from build123d import *

# Parameters (mm, degrees)
PAD_DEPTH    = 10
SKETCH001_R  = 16
POCKET_DEPTH = 3


with BuildPart() as part:
    # Sketch → Pad (new body)
    with BuildSketch(Plane.XY):
        with BuildLine():
            Line((-19, 70.33521), (19, 70.33521))
            Line((19, 70.33521), (19, -59.66479))
            ThreePointArc((-19, -59.66479), (0, -76.095918), (19, -59.66479))
            Line((-19, -59.66479), (-19, 70.33521))
        make_face()
    extrude(amount=PAD_DEPTH)

    # Sketch001 → Pocket (cut)
    with BuildSketch(Plane.XY.offset(10)):
        with Locations((0, 51.243999)):
            Circle(SKETCH001_R)
    extrude(amount=-POCKET_DEPTH, mode=Mode.SUBTRACT)


solid = part.part
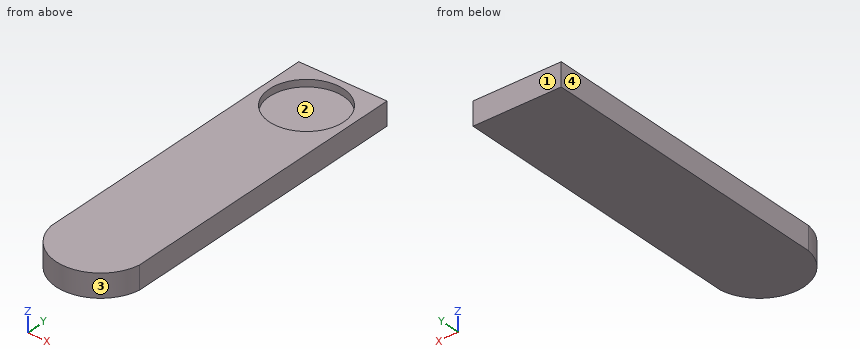
Input: part model. Units: mm. Frame: model coordinates. Face numbers are marked on the shaded views. Coordinates: 2 decimals unless noted, no trailing zeros. Loops run counter-clockwise (first coordinate to the right, second up) from the corner with the lowest first, then second, coordinate; pieces in that order, holes last. Notation, with made-up numbers: (25.25, -21.75) - (46.25, -21.75) arc R4 cw to (46.25, -16.75) - close; hole circle Ø4 at (-32.5, 33.5). An arc over 180 degrees is marked (long way). Answer in a Markdown table with one row per item. Add a question column.
Item 1: Section query B-B on y = 47. Return the cut outline in (x, z), then the cut area to 3 significant figures.
Item 2: Line query: line 1 along Y through (x, z) = (0, 8.2); line 2 along Z through (x, y) = (11, 58.5); line 3 along Y through (x, z) = (-8, 7.5). Output: solid intervals per line, ascending. Write a range as [from, to].
Item 3: Contact query for a flat-ended pin moving along its axis: P1, Ø16, axis at x = 5.5, y = 47.5, coming from the +Z side. Output: stop coordinate, or through.
Item 4: Section query A-A on x = 0. Return the cut outline in (y, z).
Item 5: Section query C-C on z = 2.5. Return the cut outline in (x, y).
Item 6: Mould query, pull axis Y, two halves, no side actions, for the marked faces 1, 2, 3 and 4. Classes: released by +Y, released by -Y, zero draft, split by the parting line, or undercut.
Recorded:
| question | item | result |
|---|---|---|
| 1 | outline | (-19, 0) - (19, 0) - (19, 10) - (15.43, 10) - (15.43, 7) - (-15.43, 7) - (-15.43, 10) - (-19, 10) - close |
| 1 | area | 287 mm^2 |
| 2 | line 1 | [-76.1, 35.24], [67.24, 70.34] |
| 2 | line 2 | [0, 7] |
| 2 | line 3 | [-74.35, 37.39], [65.1, 70.34] |
| 3 | P1 | z = 7 |
| 4 | outline | (-76.1, 0) - (70.34, 0) - (70.34, 10) - (67.24, 10) - (67.24, 7) - (35.24, 7) - (35.24, 10) - (-76.1, 10) - close |
| 5 | outline | (-19, -59.66) arc R19.2 ccw to (19, -59.66) - (19, 70.34) - (-19, 70.34) - close |
| 6 | face 1 | released by +Y |
| 6 | face 2 | undercut |
| 6 | face 3 | released by -Y |
| 6 | face 4 | zero draft |
